Build history of the part. All positions in model axes, mm. A direction names the side the tool comes from. Give positions to 0.01 mm unless a question says otherwise; leave off trailing zeros. Write each loop counter-clockwise with the first axis right and the second up, starting at its lowest first coordinate (ties: lowest second). Pieces come first, ordered by that corner, then holes.
from build123d import *

# Parameters (mm, degrees)
SKETCH1_W           = 102
SKETCH1_H           = 44
BOSS_EXTRUDE1_DEPTH = 5
CUT_EXTRUDE1_DEPTH  = 5


with BuildPart() as part:
    # Sketch1 → Boss-Extrude1 (new body)
    with BuildSketch(Plane.XY):
        Rectangle(SKETCH1_W, SKETCH1_H)
    extrude(amount=BOSS_EXTRUDE1_DEPTH)

    # Sketch3 → Cut-Extrude1 (cut)
    with BuildSketch(Plane.XY.offset(5)):
        Polygon((-36.6, 13.6), (-36.6, 8.6), (-41, 8.6), (-41, 13.6), (-42.5, 13.6), (-42.5, 17), (-41, 17), (-41, 22), (-36.6, 22), (-36.6, 17), (-35.1, 17), (-35.1, 13.6), align=None)
        Polygon((41, 8.6), (41, 13.6), (42.5, 13.6), (42.5, 17), (41, 17), (41, 22), (36.6, 22), (36.6, 17), (35.1, 17), (35.1, 13.6), (36.6, 13.6), (36.6, 8.6), align=None)
        Polygon((36.6, -13.6), (36.6, -8.6), (41, -8.6), (41, -13.6), (42.5, -13.6), (42.5, -17), (41, -17), (41, -22), (36.6, -22), (36.6, -17), (35.1, -17), (35.1, -13.6), align=None)
        Polygon((-41, -8.6), (-41, -13.6), (-42.5, -13.6), (-42.5, -17), (-41, -17), (-41, -22), (-36.6, -22), (-36.6, -17), (-35.1, -17), (-35.1, -13.6), (-36.6, -13.6), (-36.6, -8.6), align=None)
    extrude(amount=-CUT_EXTRUDE1_DEPTH, mode=Mode.SUBTRACT)


solid = part.part
(1) 3-axis set-ups, long thin cutter, end or side, ignore diameter. For faces 1 (the face through (41, 19, 3)), 2 (the face through (36.6, -20, 3)), 3 (the face through (35.1, 15, 3)): which of +Z, -Z, +X, -X, +Y, -Y reach the whole face in a straight line?
(2) Saw through at A-A, the plane y = -9.5. List the corners of the cut face in (x, z), plus the area to 3 significant figures.
(3) Mould opens along Y. For faces 4 (the face through (35.1, -15, 3)), 5 (the face through (39, 8.6, 3)), 6 (the face through (41, -19, 3)) say: +Y half, -Y half, draft (parallel to the pull), parting line (faces both ways), or undercut.
(4) Probe line 1 (X direction, y = -18, z = 1.3); line 2 (Y direction, x = -42, z = 1.25); line 3 (X direction, y = -16, z = 4.25). List the from-to ranges inside material, lowest first.
Computed values:
1. face 1: +Z, -Z, +Y
1. face 2: +Z, -Z, -Y
1. face 3: +Z, -Z
2. outline: (-51, 0) - (-41, 0) - (-41, 5) - (-51, 5) - close; (-36.6, 0) - (36.6, 0) - (36.6, 5) - (-36.6, 5) - close; (41, 0) - (51, 0) - (51, 5) - (41, 5) - close
2. area: 466 mm2
3. face 4: undercut
3. face 5: +Y half
3. face 6: draft
4. line 1: x = -51 to -41, -36.6 to 36.6, 41 to 51
4. line 2: y = -22 to -17, -13.6 to 13.6, 17 to 22
4. line 3: x = -51 to -42.5, -35.1 to 35.1, 42.5 to 51
